Build history of the part. All positions in model axes, mm. A direction names the side the tool comes from. Round coordinates to 2 decimals unless told otherwise and drop trailing zeros. Write each loop counter-clockwise with the first axis right and the second up, starting at its lowest first coordinate (ties: lowest second). Pieces come first, ordered by that corner, then holes. Notation, with made-up numbers: M 59,79.25 L 77,79.25 A32 cw 77,113.25 Z; hole C -11,86 d8. An arc over 180 degrees is marked long. Use a Markdown table: item, result.
from build123d import *

# Parameters (mm, degrees)
EXTRUDE_1_DEPTH     = 6.5
SKETCH_2_W          = 9.3
SKETCH_2_H          = 5
CUT_EXTRUDE_1_DEPTH = 14.601102896
SKETCH_3_R          = 1.75
EXTRUDE_2_DEPTH     = 2.6
SKETCH_4_W          = 13
SKETCH_4_H          = 4
SKETCH_4_W_2        = 11
SKETCH_4_H_2        = 2
EXTRUDE_3_DEPTH     = 1


with BuildPart() as part:
    # 草图1 → 凸台-拉伸1 (new, symmetric)
    with BuildSketch(Plane.XY):
        Polygon((0, 0), (9.3, 0), (9.3, 7), (-6.2, 7), (-6.2, -7.5), (0, -7.5), align=None)
    extrude(amount=EXTRUDE_1_DEPTH, both=True)

    # 草图2 → 切除-拉伸1 (cut, through all)
    with BuildSketch(Plane.XZ):
        with Locations((4.65, 0)):
            Rectangle(SKETCH_2_W, SKETCH_2_H)
    extrude(amount=-CUT_EXTRUDE_1_DEPTH, mode=Mode.SUBTRACT)

    # 草图3 → 凸台-拉伸2 (add)
    with BuildSketch(Plane.ZY.offset(6.2)):
        with BuildLine():
            Line((5.5, 14), (-5.5, 14))
            ThreePointArc((-5.5, 14), (-6.207106781, 13.707106781), (-6.5, 13))
            Line((-6.5, 13), (-6.5, 7))
            Line((-6.5, 7), (6.5, 7))
            Line((6.5, 7), (6.5, 13))
            ThreePointArc((6.5, 13), (6.207106781, 13.707106781), (5.5, 14))
        make_face()
        with Locations(Location((-3.5, 10.5, 0), (0, 0, 270))):
            Circle(SKETCH_3_R, mode=Mode.SUBTRACT)
        with Locations(Location((3.5, 10.5, 0), (0, 0, 90))):
            Circle(SKETCH_3_R, mode=Mode.SUBTRACT)
    extrude(amount=-EXTRUDE_2_DEPTH)

    # 草图4 → 凸台-拉伸3 (add)
    with BuildSketch(Plane.ZY.offset(6.2)):
        with Locations((0, -9.5)):
            Rectangle(SKETCH_4_W, SKETCH_4_H)
        with Locations((0, -9.5)):
            Rectangle(SKETCH_4_W_2, SKETCH_4_H_2, mode=Mode.SUBTRACT)
    extrude(amount=-EXTRUDE_3_DEPTH)


solid = part.part
Q1. Cut at D-D on y = 4. Give the cut face in (x, z).
Response values:
| item | result |
|---|---|
| outline | M -6.2,-6.5 L 9.3,-6.5 L 9.3,-2.5 L 0,-2.5 L 0,2.5 L 9.3,2.5 L 9.3,6.5 L -6.2,6.5 Z |
Q2. Cut at B-B on z = 3.5. Give the cut face in (x, y).
Response values:
| item | result |
|---|---|
| outline | M -6.2,-11.5 L -5.2,-11.5 L -5.2,-10.5 L -6.2,-10.5 Z; M -6.2,-8.5 L -5.2,-8.5 L -5.2,-7.5 L 0,-7.5 L 0,0 L 9.3,0 L 9.3,7 L -3.6,7 L -3.6,8.75 L -6.2,8.75 Z; M -6.2,12.25 L -3.6,12.25 L -3.6,14 L -6.2,14 Z |
Q3. Cut at A-A on x = 6. Give the cut face in (y, z), and give its area (3 significant figures).
Response values:
| item | result |
|---|---|
| outline | M 0,-6.5 L 7,-6.5 L 7,-2.5 L 0,-2.5 Z; M 0,2.5 L 7,2.5 L 7,6.5 L 0,6.5 Z |
| area | 56.0 mm2 |
Q4. Drop flat-ended pins along their axis: P1, Ø5.5, axis at y = 10.5, z = 3.5, coming from the +X side; P2, Ø6, axis at x = 5, z = 0, coming from the -Y side; P3, Ø2, axis at x = -3.5, z = 5, coming from the +Y side; P4, Ø2.5, axis at x = -2.5, z = -2, coming from the -Y side. Give the stop position or say it passes through.
Response values:
| item | result |
|---|---|
| P1 | stops at x = -3.6 |
| P2 | stops at y = 0 |
| P3 | stops at y = 14 |
| P4 | stops at y = -7.5 |
Q5. Cut at C-C on y = 10.5. Give the cut face in (x, z), and give its area (3 significant figures).
Response values:
| item | result |
|---|---|
| outline | M -6.2,-6.5 L -3.6,-6.5 L -3.6,-5.25 L -6.2,-5.25 Z; M -6.2,-1.75 L -3.6,-1.75 L -3.6,1.75 L -6.2,1.75 Z; M -6.2,5.25 L -3.6,5.25 L -3.6,6.5 L -6.2,6.5 Z |
| area | 15.6 mm2 |
Q6. Two-plate mould, pull along Y, no slides. Class faces 5 (the flat face through (0, 3, -6.5)), 6 (the flat face through (-6, -8.5, 0)), 7 (the cylindrical face through (-4.918, 13.715, -6.199)): +Y half, -Y half, draft (parallel to the pull), parting line (faces both ways), or undercut.
Response values:
| item | result |
|---|---|
| face 5 | draft |
| face 6 | undercut |
| face 7 | +Y half |
Q7. Drill centre lines: L1, parallel to Z at x = -5.6, y = 10.5; L2, parallel to Z at x = 6.75, y = 6.75; L3, parallel to Y at x = -2, z = -3.75. Where is each one in solid material? Low to high.
Response values:
| item | result |
|---|---|
| L1 | z = -6.5 to -5.25, -1.75 to 1.75, 5.25 to 6.5 |
| L2 | z = -6.5 to -2.5, 2.5 to 6.5 |
| L3 | y = -7.5 to 7 |
Q8. Which spindle directions (+Z, -Z, +X, -X, +Y, -Y) get a long thin tool onto all of the face, cutting with end or side? Do faces 1 (the flat face through (3, 7, 3)), 2 (the flat face through (-5.2, -8, 0)), 3 (the flat face through (5, 3, -2.5)), 4 (the flat face through (-6, -10, -5.5)). Say none if no direction does.
Response values:
| item | result |
|---|---|
| face 1 | +Z, -Z, +X, +Y |
| face 2 | +Z, -Z, +X, -Y |
| face 3 | +X, +Y, -Y |
| face 4 | +X, -X |
